```python
from build123d import *

# Parameters (mm, degrees)
SKETCH1_R                = 2.5
BOSS_EXTRUDE1_DEPTH      = 4
SKETCH3_R                = 5
BOSS_EXTRUDE2_DEPTH      = 2.5
BOSS_EXTRUDE3_DEPTH      = 3.5
BOSS_EXTRUDE3_DEPTH_BACK = 4
SKETCH4_R                = 5


with BuildPart() as part:
    # Sketch1 → Boss-Extrude1 (new body)
    with BuildSketch(Plane.XY):
        Circle(SKETCH1_R)
    extrude(amount=BOSS_EXTRUDE1_DEPTH)

    # Sketch3 → Boss-Extrude2 (add)
    with BuildSketch(Plane.XY.offset(4)):
        with BuildLine():
            Line((0, 10), (350, 10))
            ThreePointArc((350, 10), (360, 0), (350, -10))
            Line((350, -10), (0, -10))
            ThreePointArc((0, -10), (-10, 0), (0, 10))
        make_face()
        with Locations((350, 0)):
            Circle(SKETCH3_R, mode=Mode.SUBTRACT)
        with BuildLine():
            Line((15, 3), (110, 3))
            ThreePointArc((110, 3), (113, 0), (110, -3))
            Line((110, -3), (15, -3))
            ThreePointArc((15, -3), (12, 0), (15, 3))
        make_face(mode=Mode.SUBTRACT)
        with BuildLine():
            Line((335, 3), (240, 3))
            ThreePointArc((240, 3), (237, 0), (240, -3))
            Line((240, -3), (335, -3))
            ThreePointArc((335, -3), (338, 0), (335, 3))
        make_face(mode=Mode.SUBTRACT)
    extrude(amount=BOSS_EXTRUDE2_DEPTH)

    # Sketch4 → Boss-Extrude3 (add, two sides: drawn at the far end of the back side and taken through both)
    with BuildSketch(Plane(origin=(0, 0, 4), x_dir=(-1, 0, 0), z_dir=(0, 0, -1)).offset(-BOSS_EXTRUDE3_DEPTH_BACK)):
        with Locations((-350, 0)):
            Circle(SKETCH4_R)
    extrude(amount=BOSS_EXTRUDE3_DEPTH + BOSS_EXTRUDE3_DEPTH_BACK)


solid = part.part
```
The listing builds one solid part. Answer for the finished solid, in the listing's coordinates (mm). Give positions to 0.01 mm unless a question says otherwise; leave off trailing zeros. Order: outer loops, then holes, each group sorted by start corner. A loop starts at its lowest first (then second) coordinate and runs counter-clockwise, first axis right, second up.
Item 1: Given pin 1 Ø6 at (x, y) = (141.5, -6) entering from +Z; pin 2 Ø1.5 at (x, y) = (100.5, -3.5) entering from -Z; pin 3 Ø3 at (x, y) = (349, 0) entering from -Z, each flat-ended and moving along its own axis, determine where each tip first touches the part or whether it passes through.
From the geometry:
pin 1: stops at z = 6.5
pin 2: stops at z = 4
pin 3: stops at z = 0.5
Item 2: The part is cut by section B-B, the plane z = 2.5. Give the vertices of the cut face in (x, y).
From the geometry:
outline: circle Ø5 at (0, 0); circle Ø10 at (350, 0)
Item 3: The part is cut by section C-C, the plane x = 210. Give the vertices of the cut face in (y, z), and give its area (3 significant figures).
From the geometry:
outline: (-10, 4) - (10, 4) - (10, 6.5) - (-10, 6.5) - close
area: 50.0 mm2
Item 4: The part is cut by section A-A, the plane x = 253. Give the vertices of the cut face in (y, z), and give its area (3 significant figures).
From the geometry:
outline: (-10, 4) - (-3, 4) - (-3, 6.5) - (-10, 6.5) - close; (3, 4) - (10, 4) - (10, 6.5) - (3, 6.5) - close
area: 35.0 mm2
Item 5: Find the intervals of material crossed by probe 1 along Y at (x, z) = (313.5, 5.75); probe 2 along Z at (x, y) = (7, 0.25); probe 3 along X at (y, z) = (7.5, 4.5), in increasing order.
From the geometry:
probe 1: y = -10 to -3, 3 to 10
probe 2: z = 4 to 6.5
probe 3: x = -6.61 to 356.61
Item 6: For a pull along X with two mould halves and no side action, classify faces 1 (the face through (345.23, 1.5, 2.27)), 2 (the face through (350, 0, 0.5)), 3 (the face through (360, 0, 5)), 4 (the face through (345.23, 1.5, 7.26)) as pulls with the +X half, pulls with the -X half, needs draft (parallel to the pull), parting line crosses it, or undercut.
From the geometry:
face 1: undercut
face 2: needs draft
face 3: pulls with the +X half
face 4: parting line crosses it
